Source: CAD feature listing. Evaluate the final solid. Frame: model axes, mm. Face numbers are marked on the shaded views. A direction names the side the tool comes from. Round coordinates to 2 decimals unless told otherwise and drop trailing zeros. Order: outer loops, then holes, each group sorted by start corner. A loop starts at its lowest first (then second) coordinate and runs counter-clockwise, first axis right, second up. Notation, with made-up numbers: (77.5, 28.25) -> (122.5, 28.25) arc R18 ccw to (122.5, 42.25) -> close; hole circle Ø1 at (-26, 0). An arc over 180 degrees is marked (long way). One line per item, written item: value. Start each with the question number.
1) Mould query, pull axis X, two halves, no side actions, for the marked faces 3, 4 and 5. Classes: pulls with the +X half, pulls with the -X half, needs draft (parallel to the pull), parting line crosses it, or undercut.
2) Section C-C (y = 0.75). Return the cut outline in (x, z), and give its area (3 significant figures).
3) Section A-A (z = 8.5). State how many separate pieces and enclosed holes the cut face has, and give its area (3 significant figures).
4) Section D-D (x = 0). Return the cut outline in (y, z).
5) Ray query, L1, parallel to Z at x = 0, y = -1.1; L2, parallel to Z at x = -16.2, y = 5.5; L3, parallel to X at y = 7.25, z = -5.5. Return the intervals inside material, ascending.
6) Pin query (flat end, axial travel): P1, Ø4, axis at x = 0, z = 8, coming from the +Y side; P2, Ø3, axis at y = 5.5, z = 8.5, coming from the +X side; P3, Ø2, axis at y = 0.5, z = 8, coming from the -X side. Return the tip coordinate at first contact, or that it passes through.
7) Reachability of the marked faces 1 and 2 from +Z, -Z, +X, -X, +Y, -Y: full face, straight path, thin tool, end or side. Return the list, or none.
8) Section B-B (x = -10). Return the cut outline in (y, z), and give its area (3 significant figures).
```python
from build123d import *

# Parameters (mm, degrees)
BASE_FLANGE1_DEPTH      = 12
SKETCH5_R               = 4
SKETCH5_R_2             = 1.3
CUT_EXTRUDE1_DEPTH      = 10
SKETCH6_W               = 1.5
SKETCH6_H               = 5.6
BOSS_EXTRUDE1_DEPTH     = 3.5
CUT_EXTRUDE2_DEPTH      = 25.04391815
CUT_EXTRUDE2_DEPTH_BACK = 25.04391815
SKETCH7_R               = 1.3
FILLET1_R               = 2
SKETCH8_R               = 1.3
CUT_EXTRUDE3_DEPTH      = 10


# Sheet-metal steps are written as plain solids
with BuildPart() as part:
    # Sketch1 → Base-Flange1 (new, symmetric)
    with BuildSketch(Plane.XY):
        with BuildLine():
            Line((-15, 8.1), (-15, 2.5))
            ThreePointArc((-15, 2.5), (-14.267766953, 0.732233047), (-12.5, 0))
            Line((-12.5, 0), (12.5, 0))
            ThreePointArc((12.5, 0), (14.267766953, 0.732233047), (15, 2.5))
            Line((15, 2.5), (15, 8.1))
            Line((15, 8.1), (16.5, 8.1))
            Line((16.5, 8.1), (16.5, 2.5))
            ThreePointArc((16.5, 2.5), (15.328427125, -0.328427125), (12.5, -1.5))
            Line((12.5, -1.5), (-12.5, -1.5))
            ThreePointArc((-12.5, -1.5), (-15.328427125, -0.328427125), (-16.5, 2.5))
            Line((-16.5, 2.5), (-16.5, 8.1))
            Line((-16.5, 8.1), (-15, 8.1))
        make_face()
    extrude(amount=BASE_FLANGE1_DEPTH, both=True)

    # Sketch5 → Cut-Extrude1 (cut)
    with BuildSketch(Plane(origin=(0, 0, 0), x_dir=(1, 0, 0), z_dir=(0, 1, 0))):
        with Locations(Location((0, 0, 0), (0, 0, 180))):
            Circle(SKETCH5_R)
        with Locations(Location((0, 8, 0), (0, 0, 180))):
            Circle(SKETCH5_R_2)
        with Locations(Location((5.656854249, 5.656854249, 0), (0, 0, 180))):
            Circle(SKETCH5_R_2)
        with Locations(Location((8, 0, 0), (0, 0, 180))):
            Circle(SKETCH5_R_2)
        with Locations(Location((5.656854249, -5.656854249, 0), (0, 0, 180))):
            Circle(SKETCH5_R_2)
        with Locations(Location((0, -8, 0), (0, 0, 180))):
            Circle(SKETCH5_R_2)
        with Locations(Location((-5.656854249, -5.656854249, 0), (0, 0, 180))):
            Circle(SKETCH5_R_2)
        with Locations(Location((-8, 0, 0), (0, 0, 180))):
            Circle(SKETCH5_R_2)
        with Locations(Location((-5.656854249, 5.656854249, 0), (0, 0, 180))):
            Circle(SKETCH5_R_2)
    extrude(amount=-CUT_EXTRUDE1_DEPTH, mode=Mode.SUBTRACT)

    # Sketch6 → Boss-Extrude1 (add)
    with BuildSketch(Plane(origin=(0, 0, -12), x_dir=(-1, 0, 0), z_dir=(0, 0, -1))):
        with Locations((-15.75, 5.3)):
            Rectangle(SKETCH6_W, SKETCH6_H)
        with Locations((15.75, 5.3)):
            Rectangle(SKETCH6_W, SKETCH6_H)
    extrude(amount=BOSS_EXTRUDE1_DEPTH)

    # Sketch7 → Cut-Extrude2 (cut, two sides: drawn at the far end of the back side and taken through both)
    with BuildSketch(Plane(origin=(0, 0, 0), x_dir=(0, 0, -1), z_dir=(1, 0, 0)).offset(-CUT_EXTRUDE2_DEPTH_BACK)):
        with Locations((-8.5, 5.5)):
            Circle(SKETCH7_R)
        with Locations((-4.5, 5.5)):
            Circle(SKETCH7_R)
        with Locations((8.5, 5.5)):
            Circle(SKETCH7_R)
        with Locations((12.5, 5.5)):
            Circle(SKETCH7_R)
    extrude(amount=CUT_EXTRUDE2_DEPTH + CUT_EXTRUDE2_DEPTH_BACK, mode=Mode.SUBTRACT)

    # Fillet1
    fillet1_edges = [part.edges().sort_by_distance(p)[0] for p in [
        (15.75, 8.1, -15.5),
        (15.75, 2.5, -15.5),
        (-15.75, 8.1, -15.5),
        (-15.75, 2.5, -15.5),
        (-15.75, 8.1, 12),
        (15.75, 8.1, 12),
    ]]
    fillet(fillet1_edges, radius=FILLET1_R)

    # Sketch8 → Cut-Extrude3 (cut)
    with BuildSketch(Plane(origin=(0, 0, 0), x_dir=(1, 0, 0), z_dir=(0, 1, 0))):
        with Locations(Location((-10, 9, 0), (0, 0, 270))):
            Circle(SKETCH8_R)
        with Locations(Location((10, 9, 0), (0, 0, 270))):
            Circle(SKETCH8_R)
        with Locations(Location((-10, -9, 0), (0, 0, 270))):
            Circle(SKETCH8_R)
        with Locations(Location((10, -9, 0), (0, 0, 270))):
            Circle(SKETCH8_R)
    extrude(amount=-CUT_EXTRUDE3_DEPTH, mode=Mode.SUBTRACT)


solid = part.part
```
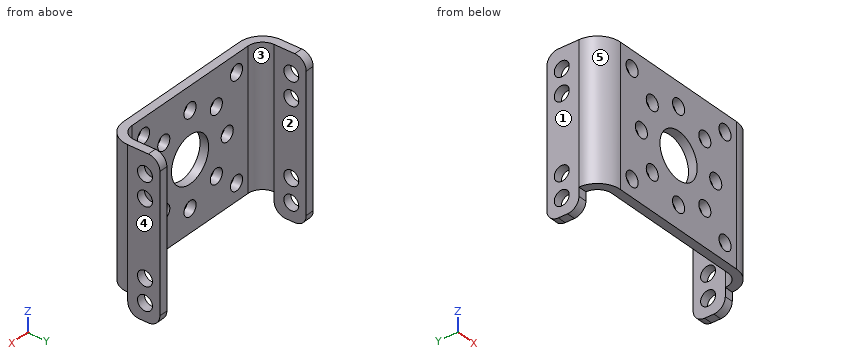
Findings:
1. face 3: undercut
1. face 4: pulls with the +X half
1. face 5: pulls with the -X half
2. outline: (-16.1, -12) -> (-14.29, -12) -> (-14.29, 12) -> (-16.1, 12) -> close; (14.29, -12) -> (16.1, -12) -> (16.1, 12) -> (14.29, 12) -> close
2. area: 87.0 mm2
3. separate pieces: 6
3. enclosed holes: 0
3. area: 51.0 mm2
4. outline: (-1.5, -12) -> (0, -12) -> (0, -9.3) -> (-1.5, -9.3) -> close; (-1.5, -6.7) -> (0, -6.7) -> (0, -4) -> (-1.5, -4) -> close; (-1.5, 4) -> (0, 4) -> (0, 6.7) -> (-1.5, 6.7) -> close; (-1.5, 9.3) -> (0, 9.3) -> (0, 12) -> (-1.5, 12) -> close
5. L1: -12 to -9.3, -6.7 to -4, 4 to 6.7, 9.3 to 12
5. L2: -15.5 to -13.8, -11.2 to -9.8, -7.2 to 3.2, 5.8 to 7.2, 9.8 to 12
5. L3: -16.5 to -15, 15 to 16.5
6. P1: y = 0
6. P2: x = 16.5
6. P3: x = -16.37
7. face 1: +Z, -Z, -X, +Y, -Y
7. face 2: +Z, -Z, +Y
8. outline: (-1.5, -12) -> (0, -12) -> (0, -10.3) -> (-1.5, -10.3) -> close; (-1.5, -7.7) -> (0, -7.7) -> (0, 7.7) -> (-1.5, 7.7) -> close; (-1.5, 10.3) -> (0, 10.3) -> (0, 12) -> (-1.5, 12) -> close
8. area: 28.2 mm2
